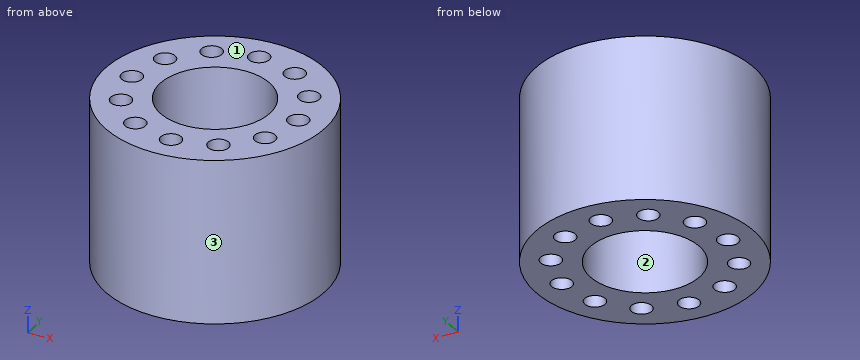
from build123d import *

# Parameters (mm, degrees)
SKETCH_1_R      = 8
SKETCH_1_R_2    = 0.75
SKETCH_1_R_3    = 4
EXTRUDE_1_DEPTH = 12


with BuildPart() as part:
    # 草图1 → 凸台-拉伸1 (new body)
    with BuildSketch(Plane.XY):
        Circle(SKETCH_1_R)
        with Locations((6, 0)):
            Circle(SKETCH_1_R_2, mode=Mode.SUBTRACT)
        with Locations((5.196152423, -3)):
            Circle(SKETCH_1_R_2, mode=Mode.SUBTRACT)
        with Locations((3, -5.196152423)):
            Circle(SKETCH_1_R_2, mode=Mode.SUBTRACT)
        with Locations((0, -6)):
            Circle(SKETCH_1_R_2, mode=Mode.SUBTRACT)
        with Locations((-3, -5.196152423)):
            Circle(SKETCH_1_R_2, mode=Mode.SUBTRACT)
        with Locations((-5.196152423, -3)):
            Circle(SKETCH_1_R_2, mode=Mode.SUBTRACT)
        with Locations((-6, 0)):
            Circle(SKETCH_1_R_2, mode=Mode.SUBTRACT)
        with Locations((-5.196152423, 3)):
            Circle(SKETCH_1_R_2, mode=Mode.SUBTRACT)
        with Locations((-3, 5.196152423)):
            Circle(SKETCH_1_R_2, mode=Mode.SUBTRACT)
        with Locations((0, 6)):
            Circle(SKETCH_1_R_2, mode=Mode.SUBTRACT)
        with Locations((3, 5.196152423)):
            Circle(SKETCH_1_R_2, mode=Mode.SUBTRACT)
        with Locations((5.196152423, 3)):
            Circle(SKETCH_1_R_2, mode=Mode.SUBTRACT)
        Circle(SKETCH_1_R_3, mode=Mode.SUBTRACT)
    extrude(amount=EXTRUDE_1_DEPTH)


solid = part.part
For this review, take the finished solid that the model builds, in its own axes (mm). Face numbers are marked on the shaded views. Round coordinates to 2 decimals unless told otherwise and drop trailing zeros. Loops run counter-clockwise (first coordinate to the right, second up) from the corner with the lowest first, then second, coordinate; pieces in that order, holes last. Notation, with made-up numbers: (26, -40) - (44, -40) arc R30 cw to (44, -18) - close; hole circle Ø1 at (-38.75, 79.5). An arc over 180 degrees is marked (long way). Use one line per item in the form item = value.
1) Clearance check with flat-ended pins moving along their axes: P1, Ø1, axis at x = -4, z = 7, coming from the +Y side; P2, Ø3, axis at y = 6.5, z = 9, coming from the +X side (3 decimals); P3, Ø5, axis at x = 6.5, z = 2, coming from the +Y side. State where each tip first meets the part, or that it passes through.
Solutions:
P1 = 7.19
P2 = 6.245
P3 = 6.93
2) We need section D-D on x = -6.5. Write out the cut boundary in (y, z).
Solutions:
outline = (-4.66, 0) - (-0.56, 0) - (-0.56, 12) - (-4.66, 12) - close; (0.56, 0) - (4.66, 0) - (4.66, 12) - (0.56, 12) - close
3) Mouldability with a two-part tool opening along X and no side actions: class the marked faces 1, 2 and 3 as pulls with the +X half, pulls with the -X half, needs draft (parallel to the pull), parting line crosses it, or undercut.
Solutions:
face_1 = needs draft
face_2 = undercut
face_3 = parting line crosses it
4) We need section C-C on z = 8.5. State how many separate pieces and enclosed holes the cut face has, then the cut area to 3 significant figures.
Solutions:
separate_pieces = 1
enclosed_holes = 13
area = 130 mm2
5) We need section A-A on y = 0. Write out the cut boundary in (x, z), then the cut area to 3 significant figures.
Solutions:
outline = (-8, 0) - (-6.75, 0) - (-6.75, 12) - (-8, 12) - close; (-5.25, 0) - (-4, 0) - (-4, 12) - (-5.25, 12) - close; (4, 0) - (5.25, 0) - (5.25, 12) - (4, 12) - close; (6.75, 0) - (8, 0) - (8, 12) - (6.75, 12) - close
area = 60.0 mm2
6) Wall thickness on probe 1 along Y at (x, z) = (0, 6.5); probe 2 along X at (y, z) = (-5.5, 4); probe 3 along Y at (x, z) = (3, 7): over which ranges is each line inside the solid? List them lowest first.
Solutions:
probe_1 = -8 to -6.75, -5.25 to -4, 4 to 5.25, 6.75 to 8
probe_2 = -5.81 to -3.69, -2.31 to -0.56, 0.56 to 2.31, 3.69 to 5.81
probe_3 = -7.42 to -5.95, -4.45 to -2.65, 2.65 to 4.45, 5.95 to 7.42
